Build history of the part. All positions in model axes, mm. A direction names the side the tool comes from. Give positions to 0.01 mm unless a question says otherwise; leave off trailing zeros. Loops run counter-clockwise (first coordinate to the right, second up) from the corner with the lowest first, then second, coordinate; pieces in that order, holes last. Notation, with made-up numbers: (32.5, -9) -> (64.5, -9) arc R27 cw to (64.5, 24) -> close; hole circle Ø3 at (46, 1.5). An arc over 180 degrees is marked (long way). One line per question, with ' | ' between items. Start each with the question number.
(1) Slice it at B-B, the plane z = 0. Write the cut outline in (x, y), then the cut area to 3 significant figures.
(2) Flat gauge pins, fed straight in: pin 1 Ø2 at (x, z) = (13.5, 13.5) entering from +Y; pin 2 Ø6.5 at (x, z) = (0, -10.66) entering from -Y. Where does each tip first touch, or does it go through?
(3) Drill centre lines: L1, parallel to Z at x = 2.5, y = -2.5; L2, parallel to X at y = -2.1, z = -4; L3, parallel to X at y = -0.8, z = 8. Where is each one in solid material? Low to high. Write a range as from..to.
(4) 3-axis set-ups, long thin cutter, end or side, ignore diameter. For faces 1 (the face through (6.646, -2.29, -12.779)), 2 (the face through (-0.438, -1.03, -12.633)): which of +Z, -Z, +X, -X, +Y, -Y reach the whole face in a straight line?
(5) Slice it at D-D, the plane y = -0.4. Give the number of separate pieces and of enclosed holes in the cut face, then the cut area to 3 significant figures.
(6) Slice it at A-A, the plane x = 0. Write the cut outline in (y, z), then the cut area to 3 significant figures.
(7) Slice it at C-C, the plane x = 11.5. Write the cut outline in (y, z), then the cut area to 3 significant figures.
(8) Mould opens along Z. For faces 3 (the face through (-1.574, -3.17, 0.069)), 4 (the face through (10.42, -1.03, 1.97)), 5 (the face through (0, 0, 0)) say: pulls with the +Z half, pulls with the -Z half, needs draft (parallel to the pull), parting line crosses it, or undercut.
```python
from build123d import *

# Parameters (mm, degrees)
F0_R      = 17.4625
F1_DEPTH  = 2.54
F2_R      = 14.4038068866
F3_DEPTH  = 0.508
F4_R      = 7.2639989676
F5_DEPTH  = 0.762
F6_R      = 1.5755390971
F7_DEPTH  = 0.762
F8_R      = 1.9006154527
F9_DEPTH  = 25.4
F10_R     = 2.0193
F11_DEPTH = 25.4
F12_R     = 1.927458399
F13_DEPTH = 25.4
F14_R     = 1.9885487684
F15_DEPTH = 25.4
F16_R     = 1.9516354427
F17_DEPTH = 25.4
F18_R     = 1.9777477245
F19_DEPTH = 25.4
F20_R     = 1.9643397756
F21_DEPTH = 25.4
F22_R     = 1.9730256653
F23_DEPTH = 25.4


# Not quite as in the source:
# - the program builds the solid bodies; features that only make, move or delete a surface that nothing else refers to are left out


with BuildPart() as f1:
    # F0 (on Front) → F1 (new body)
    with BuildSketch(Plane.XZ):
        Circle(F0_R)
    extrude(amount=F1_DEPTH)

    # F2 (on face) → F3 (cut)
    with BuildSketch(Plane.XZ.offset(2.54)):
        Circle(F2_R)
    extrude(amount=-F3_DEPTH, mode=Mode.SUBTRACT)

    # F4 (on face) → F5 (join)
    with BuildSketch(Plane.XZ.offset(2.032)):
        Circle(F4_R)
    extrude(amount=F5_DEPTH)

    # F6 (on face) → F7 (join)
    with BuildSketch(Plane.XZ.offset(2.794)):
        Circle(F6_R)
    extrude(amount=F7_DEPTH)

    # F8 (on face) → F9 (cut)
    with BuildSketch(Plane.XZ.offset(2.032)):
        with Locations((0, 10.7245491818)):
            Circle(F8_R)
    extrude(amount=-F9_DEPTH, mode=Mode.SUBTRACT)

    # F10 (on face) → F11 (cut)
    with BuildSketch(Plane.XZ.offset(2.032)):
        with Locations((0, -10.661974936)):
            Circle(F10_R)
    extrude(amount=-F11_DEPTH, mode=Mode.SUBTRACT)

    # F12 (on face) → F13 (cut)
    with BuildSketch(Plane.XZ.offset(2.032)):
        with Locations((-11.1813889816, 0)):
            Circle(F12_R)
    extrude(amount=-F13_DEPTH, mode=Mode.SUBTRACT)

    # F14 (on face) → F15 (cut)
    with BuildSketch(Plane.XZ.offset(2.032)):
        with Locations((10.6769250706, 0)):
            Circle(F14_R)
    extrude(amount=-F15_DEPTH, mode=Mode.SUBTRACT)

    # F16 (on face) → F17 (cut)
    with BuildSketch(Plane.XZ.offset(2.032)):
        with Locations((-7.8357290477, 7.4233920313)):
            Circle(F16_R)
    extrude(amount=-F17_DEPTH, mode=Mode.SUBTRACT)

    # F18 (on face) → F19 (cut)
    with BuildSketch(Plane.XZ.offset(2.032)):
        with Locations((-7.5011625886, -7.130230777)):
            Circle(F18_R)
    extrude(amount=-F19_DEPTH, mode=Mode.SUBTRACT)

    # F20 (on face) → F21 (cut)
    with BuildSketch(Plane.XZ.offset(2.032)):
        with Locations((6.8851769902, -7.5763189234)):
            Circle(F20_R)
    extrude(amount=-F21_DEPTH, mode=Mode.SUBTRACT)

    # F22 (on face) → F23 (cut)
    with BuildSketch(Plane.XZ.offset(2.032)):
        with Locations((7.1082208306, 7.200348191)):
            Circle(F22_R)
    extrude(amount=-F23_DEPTH, mode=Mode.SUBTRACT)


solid = f1.part
```
Final values:
1) outline: (-17.46, -2.54) -> (-14.4, -2.54) -> (-14.4, -2.03) -> (-13.11, -2.03) -> (-13.11, 0) -> (-17.46, 0) -> close; (-9.25, -2.03) -> (-7.26, -2.03) -> (-7.26, -2.79) -> (-1.58, -2.79) -> (-1.58, -3.56) -> (1.58, -3.56) -> (1.58, -2.79) -> (7.26, -2.79) -> (7.26, -2.03) -> (8.69, -2.03) -> (8.69, 0) -> (-9.25, 0) -> close; (12.67, -2.03) -> (14.4, -2.03) -> (14.4, -2.54) -> (17.46, -2.54) -> (17.46, 0) -> (12.67, 0) -> close | area: 71.6 mm2
2) pin 1: through | pin 2: y = -2.03
3) L1: -17.28..-14.19, -6.82..6.82, 14.19..17.28 | L2: -17..-13.84, -6.06..6.06, 13.84..17 | L3: -15.52..-9.7, -5.97..5.3, 8.91..15.52
4) face 1: -Y | face 2: +Y, -Y
5) separate pieces: 1 | enclosed holes: 8 | area: 861 mm2
6) outline: (-3.56, -1.58) -> (-2.79, -1.58) -> (-2.79, -7.26) -> (-2.03, -7.26) -> (-2.03, -8.64) -> (0, -8.64) -> (0, 8.82) -> (-2.03, 8.82) -> (-2.03, 7.26) -> (-2.79, 7.26) -> (-2.79, 1.58) -> (-3.56, 1.58) -> close; (-2.54, -17.46) -> (0, -17.46) -> (0, -12.68) -> (-2.03, -12.68) -> (-2.03, -14.4) -> (-2.54, -14.4) -> close; (-2.54, 14.4) -> (-2.03, 14.4) -> (-2.03, 12.63) -> (0, 12.63) -> (0, 17.46) -> (-2.54, 17.46) -> close | area: 71.6 mm2
7) outline: (-2.54, -13.14) -> (0, -13.14) -> (0, -1.81) -> (-2.03, -1.81) -> (-2.03, -8.67) -> (-2.54, -8.67) -> close; (-2.54, 8.67) -> (-2.03, 8.67) -> (-2.03, 1.81) -> (0, 1.81) -> (0, 13.14) -> (-2.54, 13.14) -> close | area: 50.6 mm2
8) face 3: parting line crosses it | face 4: undercut | face 5: needs draft
